Check sheet for the modelled part. Datum: model origin and axes. Units: mm. Face numbers are marked on the shaded views. A direction names the side the tool comes from. Give positions to 0.01 mm unless a question says otherwise; leave off trailing zeros. Order: outer loops, then holes, each group sorted by start corner. A loop starts at its lowest first (then second) coordinate and runs counter-clockwise, first axis right, second up.
```python
from build123d import *

# Parameters (mm, degrees)
F1_DEPTH      = 25
F2_DEPTH      = 25
F3_DEPTH      = 2
F3_DEPTH_BACK = 2
F4_R          = 5
F5_R          = 1.99999


# Not quite as in the source:
# - a fillet or chamfer is up to 0.001 mm smaller than in the source, because OpenCascade refuses the exact size


with BuildPart() as f1:
    # F0 (on Top) → F1 (new body)
    with BuildSketch(Plane.XY):
        Polygon((-40, 0), (-40, 4), (-44, 4), (-44, -60), (-40, -60), align=None)
        Polygon((0, 0), (0, 4), (-16, 4), (-40, 4), (-40, 0), align=None)
        Polygon((4, 40), (0, 40), (0, 29), (0, 4), (0, 0), (0, -40), (4, -40), align=None)
    extrude(amount=F1_DEPTH)

    # F0 (on Top) → F2 (join)
    with BuildSketch(Plane.XY):
        Polygon((4, 40), (0, 40), (0, 29), (0, 4), (0, 0), (0, -40), (4, -40), align=None)
        Polygon((0, 0), (0, 4), (-16, 4), (-40, 4), (-40, 0), align=None)
        Polygon((-40, 0), (-40, 4), (-44, 4), (-44, -60), (-40, -60), align=None)
    extrude(amount=-F2_DEPTH)

    # F0 (on Top) → F3 (join, two sides)
    with BuildSketch(Plane.XY) as f3_sk:
        Polygon((0, 4), (0, 29), (-16, 4), align=None)
    extrude(amount=F3_DEPTH)
    extrude(f3_sk.sketch, amount=-F3_DEPTH_BACK)

    # F4
    f4_edges = [f1.edges().sort_by_distance(p)[0] for p in [
        (-40, 0, 0),
        (0, 0, 0),
        (0, 4, 13.5),
        (0, 4, -13.5),
    ]]
    fillet(f4_edges, radius=F4_R)

    # F5 (radius 2 in the source; OpenCascade refuses exactly that, so slightly less here)
    f5_edges = [f1.edges().sort_by_distance(p)[0] for p in [
        (-44, 4, 0),
        (0, 40, 0),
        (-44, -60, 0),
        (-40, -60, 0),
        (0, -40, 0),
        (-16, 4, 0),
        (0, 29, 0),
    ]]
    fillet(f5_edges, radius=F5_R)


solid = f1.part
```
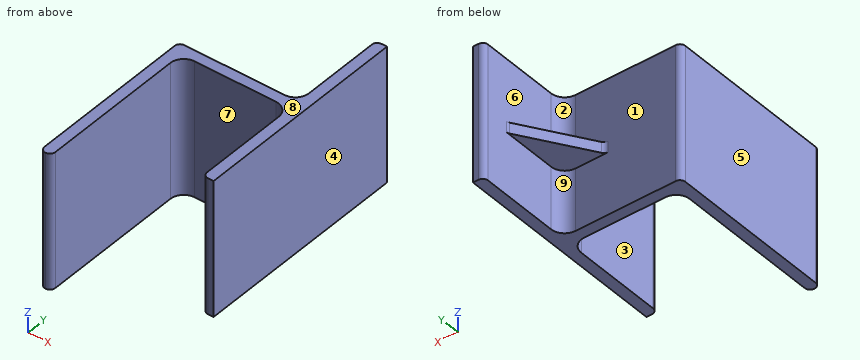
(1) Set-up check for the marked faces 5, 6, 7, 8 and 9: record each of +Z, -Z, +X, -X, +Y, -Y from which the full face is reachable in a straight line by a thin tool's end or side.
Response values:
face 5: +Z, -Z, -X, +Y, -Y
face 6: -X, +Y
face 7: +Z, -Z, -Y
face 8: +Z, +X, -X, +Y, -Y
face 9: -Z, -X, +Y
(2) Gauge pin test, flat ends, axial feed: pin 1 Ø2 at (x, z) = (2.5, 10.5) entering from -Y; pin 2 Ø24 at (x, z) = (-15, 10) entering from -Y; pin 3 Ø10 at (x, z) = (-20, -10) entering from +Y. Record the tip position at first contact, or that the pin passes through.
Response values:
pin 1: stops at y = -40
pin 2: stops at y = -0.42
pin 3: stops at y = 4
(3) Release check for a two-part mould opening along X. For the marked faces 1, 2, 3 and 4 record: released by +X, released by -X, zero draft, split by the parting line, or undercut.
Response values:
face 1: zero draft
face 2: released by -X
face 3: undercut
face 4: released by +X
(4) Cross-section at C-C on y = 20.5. Enter the section's corners in (x, z), then the cut area to 3 significant figures.
Response values:
outline: (-5.44, -2) - (0, -2) - (0, -25) - (4, -25) - (4, 25) - (0, 25) - (0, 2) - (-5.44, 2) - close
area: 222 mm2
(5) Cross-section at A-A on y = -10.5. Enter the section's corners in (x, z).
Response values:
outline: (-44, -25) - (-40, -25) - (-40, 25) - (-44, 25) - close; (0, -25) - (4, -25) - (4, 25) - (0, 25) - close
(6) Material ranges on L1, parallel to X at y = -9, z = -7; L2, parallel to X at y = 33, z = -22, recorded low to high.
Response values:
L1: x = -44 to -40, 0 to 4
L2: x = 0 to 4
(7) Cross-section at D-D on x = -12.5. Enter the section's corners in (y, z), then the cut area to 3 significant figures.
Response values:
outline: (0, -25) - (4, -25) - (4, -2) - (9.47, -2) - (9.47, 2) - (4, 2) - (4, 25) - (0, 25) - close
area: 222 mm2
